Autodesk Inventor part; units mm, degrees
ref_plane "Work Plane3" through (0, -2, -2) normal (0, 0, -1) x (-1, 0, 0)
ref_plane "Work Plane4" through (0, 15.5, 120) normal (0, -1, 0) x (0, 0, -1)
ref_plane "YZ Plane" through (0, 0, 0) normal (1, 0, 0) x (0, 1, 0)
ref_plane "Work Plane3" through (0, -2, -2) normal (0, 0, -1) x (-1, 0, 0)
sketch "Sketch4" plane through (0, -2, -2) normal (0, 0, -1) x (-1, 0, 0)
  line L0 (-30, 2) -> (-30, 3)
  line L1 (3, -2) -> (-26, -2)
  line L2 (7, 2) -> (7, 33)
  line L3 (3, 37) -> (-26, 37)
  line L4 (-27, 17.5) -> (-42, 17.5)
  line L5 (-30, 3.2) -> (-26, 0.2)
  line L6 (-26.2, 0.2) -> (-26.2, 17.5)
  line L7 (-30, 3.2) -> (-30, 17.5)
  line L8 (-30, 31.8) -> (-26, 34.8)
  line L9 (-26.2, 34.8) -> (-26.2, 17.5)
  line L10 (-30, 31.8) -> (-30, 17.5)
  arc A0 (3, -2) -> (7, 2) centre (3, 2) ccw
  arc A1 (7, 33) -> (3, 37) centre (3, 33) ccw
  arc A2 (-26, 37) -> (-30, 33) centre (-26, 33) ccw
  arc A3 (-30, 2) -> (-26, -2) centre (-26, 2) ccw
  line L11 (-30, 32) -> (-30, 33)
  line L12 (-26, 35) -> (-26, 0)
  line L13 (-26, 0) -> (-30, 3)
  line L14 (-26.2, 3.2) -> (-25.2, 3.2)
  line L15 (-25.2, 3.2) -> (-25.2, 17.5)
  line L16 (-26.2, 31.8) -> (-25.2, 31.8)
  line L17 (-25.2, 31.8) -> (-25.2, 17.5)
  line L18 (-30, 32) -> (-26, 35)
  circle A4 centre (-11.5, 17.5) radius 8
  point P0 (0, 2)
  point P1 (-26.2, 0.35)
  point P2 (-26.2, 34.65)
  point P3 (-26.2, 31.8)
  dimension "d55" = 1
  dimension "d56" = 4
  dimension "d57" = 3
  dimension "d58" = 0.2
  dimension "d59" = 3.8
extrude "Whole Cover" add sketch "Sketch4" against normal blind 122 contours L5 L7 L10 L8 L9 L6
ref_plane "Work Plane4" through (0, 15.5, 120) normal (0, -1, 0) x (0, 0, -1)
sketch "Sketch5" plane through (0, 15.5, 120) normal (0, -1, 0) x (0, 0, -1)
  line L0 (122, 30) -> (0, 30)
  line L1 (122, 26.2) -> (0, 26.2)
  line L2 (0, 26.2) -> (0, 30)
  line L3 (7.85, 30) -> (-0.75, 30)
  line L4 (3.55, 30) -> (3.55, 27.8)
  line L5 (3.0945, 28.033) -> (-0.75, 30)
  line L6 (4.0055, 28.033) -> (7.85, 30)
  arc A0 (3.0945, 28.033) -> (4.0055, 28.033) centre (3.55, 28.9233) ccw
  point P0 (120, 0)
  point P1 (0, 29.6163)
  point P2 (0, 30)
  dimension "d45" = 8.6
  dimension "d47" = 2.2
  dimension "d48" = 1
extrude "Snap fit" cut sketch "Sketch5" along normal through all both and the other way through all
sketch "Sketch6" plane through (30, 1.2, -2) normal (1, 0, 0) x (0, 0, -1)
  line L0 (0, -2.85) -> (0, 31.45)
  line L1 (0, 14.3) -> (-7, 14.3) construction
  line L2 (-7, 9.3) -> (-10, 9.3)
  line L3 (-10, 9.3) -> (-10, 19.3)
  line L4 (-10, 19.3) -> (-7, 19.3)
  line L5 (-7, 19.3) -> (-7, 9.3)
  point P0 (-2, -1.2)
  dimension "d15" = 3
  dimension "d16" = 10
  dimension "d17" = 7
extrude "Grip" cut sketch "Sketch6" against normal blind 2
chamfer "Grip Chamfer" distance 1.5 angle 45 2 edges at (28, 15.5, 8) (28, 15.5, 5)
sketch "Sketch9" plane through (30, 1.2, -2) normal (1, 0, 0) x (0, 0, -1)
  line L0 (0, 0) -> (-122, 0)
  line L1 (-122, 31.45) -> (-122, -2.85)
  line L2 (-122, 14.3) -> (-114.6731, 14.3)
  line L3 (0, -2.85) -> (-122, -2.85)
  line L4 (-122, -2.85) -> (-114.5, -2.85)
  line L5 (-114.5, -2.85) -> (-114.5, 0.15)
  line L6 (-114.5, 0.15) -> (-122, 0.15)
  line L7 (-122, 0.15) -> (-122, -2.85)
  line L8 (-122, 31.45) -> (-114.5, 31.45)
  line L9 (-114.5, 31.45) -> (-114.5, 28.45)
  line L10 (-114.5, 28.45) -> (-122, 28.45)
  line L11 (-122, 28.45) -> (-122, 31.45)
  line L12 (-122, 28.45) -> (-121.8, 28.45)
  line L13 (-121.8, 28.45) -> (-121.8, 0.15)
  line L14 (-121.8, 0.15) -> (-122, 0.15)
  line L15 (-122, 0.15) -> (-122, 28.45)
  line L16 (-117.25, 0.15) -> (-117.25, -2.85)
  line L17 (-117.25, 28.45) -> (-117.25, 31.45)
  line L18 (-114.5, 9.3) -> (-122.5, 9.3)
  line L19 (-122.5, 9.3) -> (-122.5, 19.3)
  line L20 (-122.5, 19.3) -> (-114.5, 19.3)
  line L21 (-114.5, 19.3) -> (-114.5, 9.3)
  line L22 (-114.5, 0.15) -> (-114.5, 9.3)
  line L23 (-114.5, 19.3) -> (-114.5, 28.45)
  point P0 (-2, -1.2)
  point P1 (-117.25, 0)
  point P2 (-117.25, 28.6)
  point P3 (-122, 28.6)
  point P4 (-117.25, 0)
  point P5 (-114.5, 0)
  point P6 (-121.8, 9.3)
  point P7 (-121.8, 19.3)
  dimension "d41" = 7.5
  dimension "d42" = 3
  dimension "d43" = 0.2
  dimension "d44" = 2.75
  dimension "d49" = 8
  dimension "d50" = 10
extrude "Corner Cut" cut sketch "Sketch9" against normal through all contours L5 L3 L16 L0 | L0 L16 L6 L5 | L16 L3 L1 L0 | L0 L1 L6 L16 | L6 L13 L18 L22 | L1 L18 L13 L6 | L18 L1 L2 L13 | L20 L13 L10 L23 | L2 L1 L20 L13 | L20 L1 L10 L13 | L10 L17 L8 L9 | L10 L1 L8 L17
fillet "Fillet5" radius 1 1 edges at (29.514, 15.5, 119.8)
properties part number "enclosure cover_3DPrint"
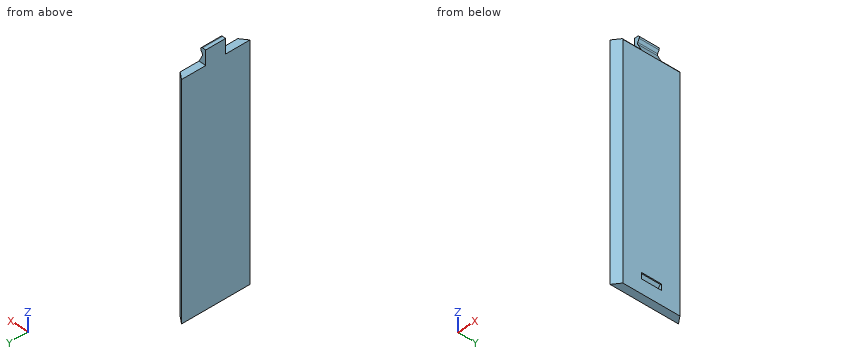
Could you check a few things on this model? Use its own coordinates, in mm. Round coordinates to 2 decimals unless told otherwise and drop trailing zeros. Order: outer loops, then holes, each group sorted by start corner. A loop starts at its lowest first (then second) coordinate and runs counter-clockwise, first axis right, second up. Notation, with made-up numbers: (87.25, -39) -> (105.25, -39) arc R32 ccw to (105.25, -5) -> close; hole circle Ø5 at (-30, 33). An arc over 180 degrees is marked (long way). One line per question, with ' | ' between items.
Q1. I'm going to push flat-ended pins straight in: pin 1 (1 mm diameter, centred on x = 27, z = 71, fed in from +Y) (3 decimals); pin 2 (1.6 mm diameter, centred on x = 29, z = 6, fed in from -Y); pin 3 (1.8 mm diameter, centred on x = 28.5, z = 117, fed in from +Y). Where does each tip first touch, or does it pass through?
Computed values:
pin 1: y = 32.425 | pin 2: y = -0.15 | pin 3: y = 20.5
Q2. If I drill on line 1 (Z direction, x = 29.75, y = 7); line 2 (Z direction, x = 28.45, y = 14.5); line 3 (Z direction, x = 29.35, y = 17), over which ranges is the centre line in solid material (lowest first)? Write a range as from..to.
Computed values:
line 1: -2..112.5 | line 2: -2..6.05, 6.95..115.18, 117.72..119.62 | line 3: -2..5.15, 7.85..113.42
Q3. If we section it at B-B on z = 81: Write out the boundary of the cut face in (x, y), plus the area to 3 significant figures.
Computed values:
outline: (26.2, -1.65) -> (30, 1.2) -> (30, 29.8) -> (26.2, 32.65) -> close | area: 120 mm²
Q4. If we section it at A-A on y = 25: Write out the boundary of the cut face in (x, z), plus the area to 3 significant figures.
Computed values:
outline: (26.2, -2) -> (30, -2) -> (30, 112.15) -> (29.82, 112.5) -> (26.2, 112.5) -> close | area: 435 mm²
